from build123d import *

# Parameters (mm, degrees)
ESQUISSE1_R          = 1.75
BASE_EXTRUSION_DEPTH = 10


with BuildPart() as part:
    # Esquisse1 → Base-Extrusion (new body)
    with BuildSketch(Plane.XY):
        with BuildLine():
            Line((3, 0), (24.7, 0))
            ThreePointArc((24.7, 0), (24.912132034, -0.087867966), (25, -0.3))
            Line((25, -0.3), (25, -0.7))
            ThreePointArc((25, -0.7), (24.912132034, -0.912132034), (24.7, -1))
            Line((24.7, -1), (3.3, -1))
            ThreePointArc((3.3, -1), (3.087867966, -1.087867966), (3, -1.3))
            Line((3, -1.3), (3, -2.7))
            ThreePointArc((3, -2.7), (3.087867966, -2.912132034), (3.3, -3))
            Line((3.3, -3), (3.7, -3))
            ThreePointArc((3.7, -3), (3.912132034, -2.912132034), (4, -2.7))
            Line((4, -2.7), (4, -1.8))
            ThreePointArc((4, -1.8), (4.087867966, -1.587867966), (4.3, -1.5))
            Line((4.3, -1.5), (25.7, -1.5))
            ThreePointArc((25.7, -1.5), (25.912132034, -1.412132034), (26, -1.2))
            Line((26, -1.2), (26, 0.2))
            ThreePointArc((26, 0.2), (26.087867966, 0.412132034), (26.3, 0.5))
            Line((26.3, 0.5), (27, 0.5))
            ThreePointArc((27, 0.5), (29.121320344, 1.378679656), (30, 3.5))
            Line((30, 3.5), (30, 13))
            ThreePointArc((30, 13), (29.121320344, 15.121320344), (27, 16))
            Line((27, 16), (3, 16))
            ThreePointArc((3, 16), (0.878679656, 15.121320344), (0, 13))
            Line((0, 13), (0, 3))
            ThreePointArc((0, 3), (0.878679656, 0.878679656), (3, 0))
        make_face()
        with Locations((3, 13)):
            Circle(ESQUISSE1_R, mode=Mode.SUBTRACT)
        with Locations((27, 3.5)):
            Circle(ESQUISSE1_R, mode=Mode.SUBTRACT)
    extrude(amount=BASE_EXTRUSION_DEPTH)


solid = part.part
The model under review builds one solid part; all positions refer to its coordinate system, in mm. A direction names the side the tool comes from. Give positions to 0.01 mm unless a question says otherwise; leave off trailing zeros. Write each loop counter-clockwise with the first axis right and the second up, starting at its lowest first coordinate (ties: lowest second). Pieces come first, ordered by that corner, then holes.
1. Add section C-C, the plane y = 14. Write out the cut boundary in (x, z).
2. Wall thickness on L1, parallel to Y at x = 27, z = 7.25; L2, parallel to Y at x = 14.5, z = 6.75; L3, parallel to X at y = -1.75, z = 4.5: over which ranges is each line inside the solid? List them lowest first.
3. For P1, Ø1, axis at x = 5.5, z = 3, coming from the -Y side; P2, Ø1.5, axis at y = -0.5, z = 5, coming from the +X side; P3, Ø1, axis at y = -2.5, z = 7.5, coming from the +X side, all flat-tipped, find the tip position at first contact; note any pin that passes through.
4. Draft analysis for pull direction Y (two halves, no side actions). For faces 4 (the cylindrical face through (0.86, 0.9, 4.93)), 5 (the flat face through (15, 9, 10)), 6 (the cylindrical face through (0.9, 15.14, 4.93)), 7 (the flat face through (14, 0, 5)), state which applies: +Y half, -Y half, draft (parallel to the pull), parting line (faces both ways), or undercut.
5. Add section D-D, the plane y = 1. Write out the cut boundary in (x, z).
6. Add section B-B, the plane z = 8.25. Write out the cut boundary in (x, y).
7. Add section A-A, the plane x = 16.75. Write out the cut boundary in (y, z), plus the area to 3 significant figures.
8. Tool access review of faces 1 (the flat face through (26, -1, 5)), 2 (the flat face through (14, -1, 5)), 3 (the flat face through (3, -2, 5)): name each direction out of +Z, -Z, +X, -X, +Y, -Y from which nothing blocks a thin tool from reaching the whole face with its end or side.
Worked answers:
1. outline: (0.17, 0) - (1.56, 0) - (1.56, 10) - (0.17, 10) - close; (4.44, 0) - (29.83, 0) - (29.83, 10) - (4.44, 10) - close
2. L1: y = 0.5 to 1.75, 5.25 to 16
2. L2: y = -1.5 to -1, 0 to 16
2. L3: x = 3 to 4
3. P1: stops at y = -1.5
3. P2: stops at x = 26
3. P3: stops at x = 4
4. face 4: -Y half
4. face 5: draft
4. face 6: +Y half
4. face 7: undercut
5. outline: (0.76, 0) - (28.66, 0) - (28.66, 10) - (0.76, 10) - close
6. outline: (0, 3) arc R3 ccw to (3, 0) - (24.7, 0) arc R0.3 cw to (25, -0.3) - (25, -0.7) arc R0.3 cw to (24.7, -1) - (3.3, -1) arc R0.3 ccw to (3, -1.3) - (3, -2.7) arc R0.3 ccw to (3.3, -3) - (3.7, -3) arc R0.3 ccw to (4, -2.7) - (4, -1.8) arc R0.3 cw to (4.3, -1.5) - (25.7, -1.5) arc R0.3 ccw to (26, -1.2) - (26, 0.2) arc R0.3 cw to (26.3, 0.5) - (27, 0.5) arc R3 ccw to (30, 3.5) - (30, 13) arc R3 ccw to (27, 16) - (3, 16) arc R3 ccw to (0, 13) - close; hole circle Ø3.5 at (3, 13); hole circle Ø3.5 at (27, 3.5)
7. outline: (-1.5, 0) - (-1, 0) - (-1, 10) - (-1.5, 10) - close; (0, 0) - (16, 0) - (16, 10) - (0, 10) - close
7. area: 165 mm2
8. face 1: +Z, -Z, +X, -Y
8. face 2: +Z, -Z, -X
8. face 3: +Z, -Z, -X, -Y
